Check sheet for the drawn part. Datum: minimum x, y, z corner. Units: mm. Give positions to 0.01 mm unless a question says otherwise; leave off trailing zeros. Order: outer loops, then holes, each group sorted by start corner. A loop starts at its lowest first (then second) coordinate and runs counter-clockwise, first axis right, second up. Notation, with made-up numbers: (67.25, 56) -> (78.25, 56) arc R24 ccw to (78.25, 76) -> close; hole circle Ø11 at (26, 5.5). An arc over 180 degrees is marked (long way). Answer in a Markdown table with one row per item. Add a question column.
(1) Cross-section at B-B (x = 100). Record the cut outline in (y, z), then the cut area to 3 significant figures.
(2) Cross-section at C-C (z = 100). Record the cut outline in (x, y), then the cut area to 3 significant figures.
(3) Cross-section at A-A (z = 180). Record the cut outline in (x, y), then the cut area to 3 significant figures.
(4) Thickness scan on L1, parallel to Z at x = 180, y = 102.9; L2, parallel to Z at x = 100, y = 38. Record the ranges inside material, lowest first. Write a range as [from, to].
(5) Cross-section at D-D (y = 80). Record the cut outline in (x, z), then the cut area to 3 significant figures.
(6) Release check for a two-part mould opening along X. For the marked faces 1, 2 and 3 record: released by +X, released by -X, zero draft, split by the parting line, or undercut.
(7) Go/stop test with flat-tipped pins: pin 1 (2 mm diameter, centred on y = 71, z = 115.5, fed in from -X); pin 2 (14 mm diameter, centred on x = 100, y = 80, fed in from -Z); pin 3 (12 mm diameter, centred on x = 120, z = 36, fed in from -Y). Record where each tip stops, or that it passes through.
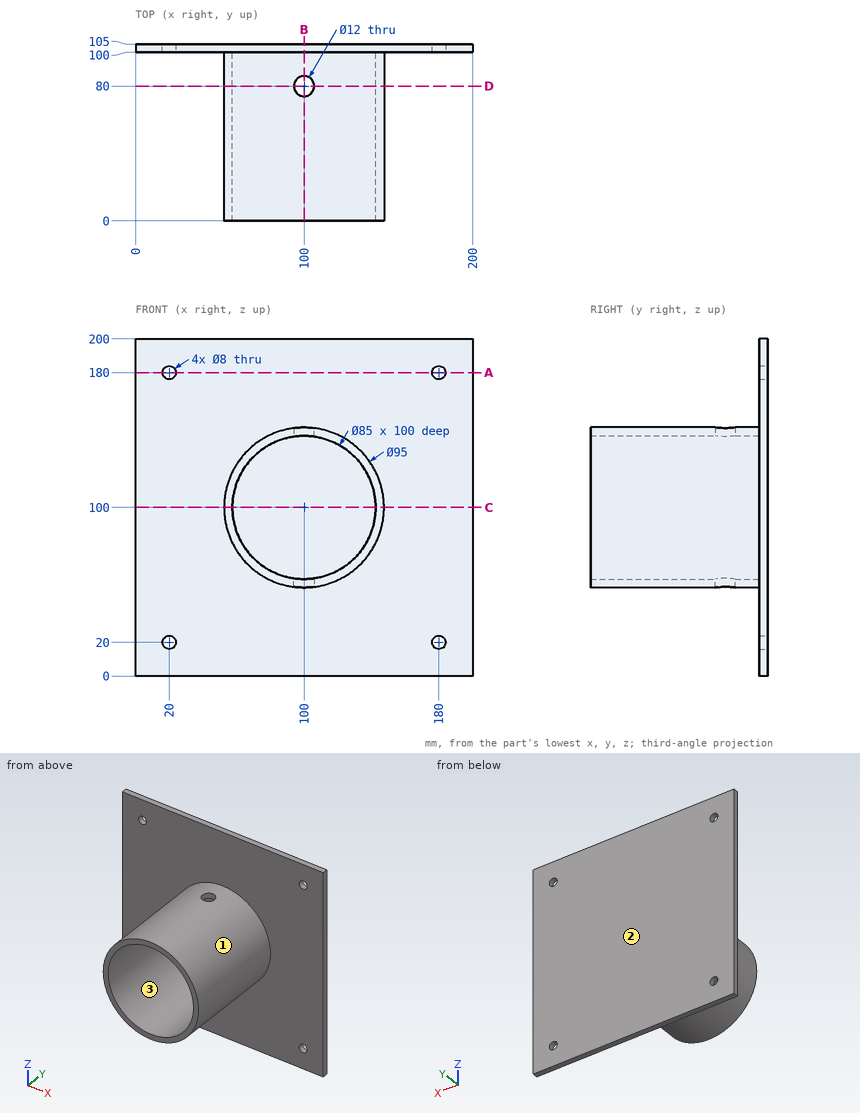
Answer below:
| question | item | result |
|---|---|---|
| 1 | outline | (0, 52.5) -> (74, 52.5) -> (74, 57.5) -> (0, 57.5) -> close; (0, 142.5) -> (74, 142.5) -> (74, 147.5) -> (0, 147.5) -> close; (86, 52.5) -> (100, 52.5) -> (100, 0) -> (105, 0) -> (105, 200) -> (100, 200) -> (100, 147.5) -> (86, 147.5) -> (86, 142.5) -> (100, 142.5) -> (100, 57.5) -> (86, 57.5) -> close |
| 1 | area | 1,880 mm² |
| 2 | outline | (0, 100) -> (52.5, 100) -> (52.5, 0) -> (57.5, 0) -> (57.5, 100) -> (142.5, 100) -> (142.5, 0) -> (147.5, 0) -> (147.5, 100) -> (200, 100) -> (200, 105) -> (0, 105) -> close |
| 2 | area | 2,000 mm² |
| 3 | outline | (0, 100) -> (16, 100) -> (16, 105) -> (0, 105) -> close; (24, 100) -> (176, 100) -> (176, 105) -> (24, 105) -> close; (184, 100) -> (200, 100) -> (200, 105) -> (184, 105) -> close |
| 3 | area | 920 mm² |
| 4 | L1 | z = [0, 16], [24, 176], [184, 200] |
| 4 | L2 | z = [52.5, 57.5], [142.5, 147.5] |
| 5 | outline | (94, 52.88) -> (94, 57.93) arc R42.5 cw to (94, 142.07) -> (94, 147.12) arc R47.5 ccw to start; (106, 52.88) arc R47.5 ccw to (106, 147.12) -> (106, 142.07) arc R42.5 cw to (106, 57.93) -> close |
| 5 | area | 1,290 mm² |
| 6 | face 1 | split by the parting line |
| 6 | face 2 | zero draft |
| 6 | face 3 | undercut |
| 7 | pin 1 | stops at x = 54.77 |
| 7 | pin 2 | stops at z = 52.5 |
| 7 | pin 3 | stops at y = 100 |
